Geometry check sheet. Reference: drawing and pictorial views, mm from the part's lowest x, y, z. Give positions to 0.01 mm unless a question says otherwise; leave off trailing zeros. Loops run counter-clockwise (first coordinate to the right, second up) from the corner with the lowest first, then second, coordinate; pieces in that order, holes last. Notation, with made-up numbers: (-33.5, 27.25) -> (9.5, 27.25) arc R22 ccw to (9.5, 49.25) -> close; hole circle Ø2 at (2, 50.25). An arc over 180 degrees is marked (long way). One line per item, written item: value. Start each with the question number.
(1) Sectioned sample at B-B, the plane y = 27.5. State how many separate pieces and enclosed holes the cut face has, then the cut area to 3 significant figures.
(2) Gauge pin test, flat ends, axial feed: pin 1 Ø7 at (x, y) = (3.5, 7.5) entering from -Z; pin 2 Ø2 at (x, y) = (28, 21) entering from -Z; pin 3 Ø2 at (x, y) = (96.5, 27.5) entering from +Z; pin 4 Ø1.8 at (x, y) = (2, 28) entering from +Z. Record the tip position at first contact, or that the pin passes through.
(3) Sectioned sample at A-A, the plane x = 3.5. Record the cut outline in (y, z).
(4) Scan lines: line 1 along Y through (x, z) = (76.5, 2.9); line 2 along Y through (x, z) = (96.5, 1.4); line 3 along X through (y, z) = (24, 1.75). Record each from-to range of solid material in increasing order. Write a range as from..to.
(5) Sectioned sample at D-D, the plane x = 76.5. Record the cut outline in (y, z), then the cut area to 4 significant figures.
(6) Draft check along X on the marked faces 1 and 2. Enter one of: pulls with the +X half, pulls with the -X half, needs draft (parallel to the pull), parting line crosses it, or undercut.
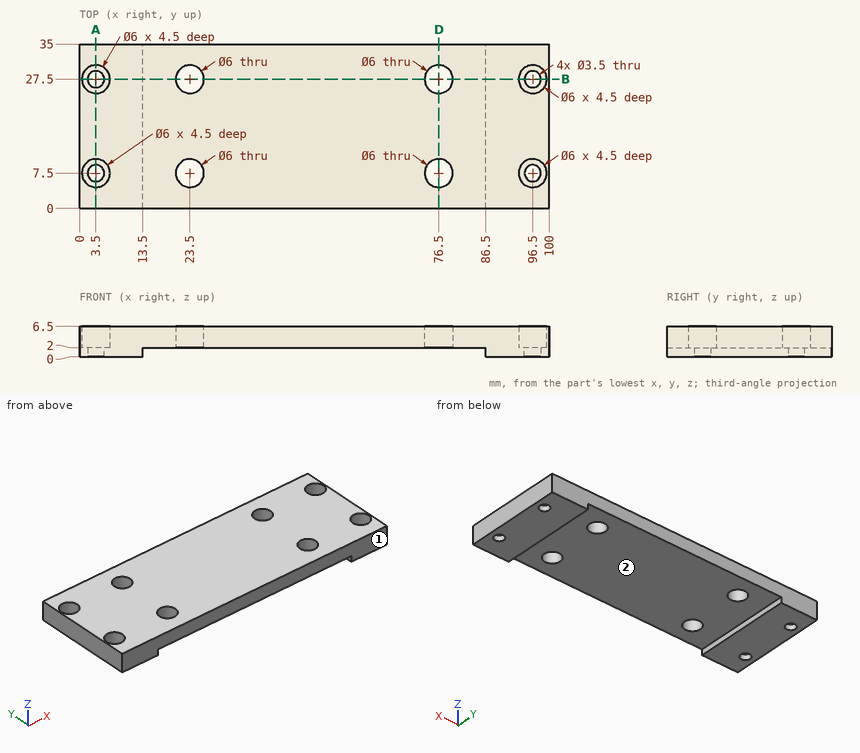
Calculated:
1. separate pieces: 5
1. enclosed holes: 0
1. area: 382 mm2
2. pin 1: stops at z = 0
2. pin 2: stops at z = 2
2. pin 3: passes through
2. pin 4: stops at z = 2
3. outline: (0, 0) -> (5.75, 0) -> (5.75, 2) -> (4.5, 2) -> (4.5, 6.5) -> (0, 6.5) -> close; (9.25, 0) -> (25.75, 0) -> (25.75, 2) -> (24.5, 2) -> (24.5, 6.5) -> (10.5, 6.5) -> (10.5, 2) -> (9.25, 2) -> close; (29.25, 0) -> (35, 0) -> (35, 6.5) -> (30.5, 6.5) -> (30.5, 2) -> (29.25, 2) -> close
4. line 1: y = 0..4.5, 10.5..24.5, 30.5..35
4. line 2: y = 0..5.75, 9.25..25.75, 29.25..35
4. line 3: x = 0..13.5, 86.5..100
5. outline: (0, 2) -> (4.5, 2) -> (4.5, 6.5) -> (0, 6.5) -> close; (10.5, 2) -> (24.5, 2) -> (24.5, 6.5) -> (10.5, 6.5) -> close; (30.5, 2) -> (35, 2) -> (35, 6.5) -> (30.5, 6.5) -> close
5. area: 103.5 mm2
6. face 1: needs draft
6. face 2: undercut
